Build history of the part. All positions in model axes, mm. A direction names the side the tool comes from. Coordinates: 2 decimals unless noted, no trailing zeros. Write each loop counter-clockwise with the first axis right and the second up, starting at its lowest first coordinate (ties: lowest second). Pieces come first, ordered by that corner, then holes.
Autodesk Inventor part; units mm, degrees
ref_plane "YZ Plane" through (0, 0, 0) normal (1, 0, 0) x (0, 1, 0)
ref_plane "XZ Plane" through (0, 0, 0) normal (0, 1, 0) x (-1, 0, 0)
ref_plane "XY Plane" through (0, 0, 0) normal (0, 0, 1) x (1, 0, 0)
sketch "Sketch1" plane through (0, 0, 0) normal (0, 1, 0) x (-1, 0, 0)
  circle A0 centre (0, 0) radius 4
  line L0 (6, 13) -> (4, 13)
  line L1 (6, -13) -> (4, -13)
  arc A1 (4, 4.4721) -> (4, -4.4721) centre (0, 0) ccw
  line L2 (4, 13) -> (4, 4.4721)
  line L3 (4, -4.4721) -> (4, -13)
  line L4 (6, 13) -> (6, -13)
  dimension "d0" = 8
  dimension "d2" = 26
  dimension "d3" = 2
extrude "Extrusion1" add sketch "Sketch1" along normal blind 16
sketch "Sketch2" plane through (-6, 0, -13) normal (-1, 0, 0) x (0, 0, 1)
  circle A0 centre (3.35, 13.6) radius 1.6
  circle A1 centre (22.65, 13.6) radius 1.6
  line L0 (8.5279, 16) -> (0, 16)
  line L1 (0, 16) -> (26, 16)
  point P0 (13, 0)
  dimension "d10" = 3.2
  dimension "d11" = 3.2
  dimension "d14" = 2.4
  dimension "d15" = 2.4
extrude "Extrusion2" cut sketch "Sketch2" against normal blind 16
properties part number "Support endStop v1"
1. Saw through at D-D on y = 10.25. List the corners of the cut face in (x, z), plus the area to 3 significant figures.
Computed values:
outline: (-6, -13) - (-4, -13) - (-4, -4.47) arc R6 ccw (long way) to (-4, 4.47) - (-4, 13) - (-6, 13) - close; hole circle Ø8 at (0, 0)
area: 102 mm2
2. Probe line 1 along Y through (x, z) = (-4.45, -9.65); line 2 along Z through (x, y) = (-1.25, 11.5); line 3 along Z through (x, y) = (1.5, 10.25). List the from-to ranges inside material, lowest first.
Computed values:
line 1: y = 0 to 12, 15.2 to 16
line 2: z = -5.87 to -3.8, 3.8 to 5.87
line 3: z = -5.81 to -3.71, 3.71 to 5.81
3. Mould opens along Z. For faces 1 (the face through (-5.01, 13.67, -11.25)), 2 (the face through (-5, 8, 13)), 3 (the face through (-4, 8, -9)) say: +Z half, -Z half, draft (parallel to the pull), parting line (faces both ways), or undercut.
Computed values:
face 1: undercut
face 2: +Z half
face 3: draft
4. Saw through at B-B on z = 9.65. List the corners of the cut face in (x, y).
Computed values:
outline: (-6, 0) - (-4, 0) - (-4, 12) - (-6, 12) - close; (-6, 15.2) - (-4, 15.2) - (-4, 16) - (-6, 16) - close
5. Saw through at A-A on y = 13.6. List the corners of the cut face in (x, z), plus the area to 3 significant figures.
Computed values:
outline: (-6, -13) - (-4, -13) - (-4, -11.25) - (-6, -11.25) - close; (-6, -8.05) - (-4, -8.05) - (-4, -4.47) arc R6 ccw (long way) to (-4, 4.47) - (-4, 8.05) - (-6, 8.05) - close; (-6, 11.25) - (-4, 11.25) - (-4, 13) - (-6, 13) - close; hole circle Ø8 at (0, 0)
area: 89.6 mm2
6. Saw through at C-C on x = 0. List the corners of the cut face in (y, z).
Computed values:
outline: (0, -6) - (16, -6) - (16, -4) - (0, -4) - close; (0, 4) - (16, 4) - (16, 6) - (0, 6) - close
7. 3-axis set-ups, long thin cutter, end or side, ignore diameter. For faces 4 (the face through (-4, 8, 9)), 5 (the face through (-5.014, 15.186, 9.442)): which of +Z, -Z, +X, -X, +Y, -Y reach the whole face in a straight line?
Computed values:
face 4: +Z, +Y, -Y
face 5: +X, -X
8. Flat gauge pins, fed straight in: pin 1 (1 mm diameter, centred on x = -3, y = 8, fed in from +Z); pin 2 (3.5 mm diameter, centred on y = 13.6, z = -9.65, fed in from +X); pin 3 (1.9 mm diameter, centred on y = 13.6, z = 9.65, fed in from -X); pin 4 (6 mm diameter, centred on x = 4, y = 11, fed in from +Z). Where does each tip first touch, or does it go through?
Computed values:
pin 1: stops at z = 5.45
pin 2: stops at x = -4
pin 3: passes through
pin 4: stops at z = 5.92
